from build123d import *

# Parameters (mm, degrees)
BOSS_EXTRUDE1_DEPTH = 9.525
SKETCH3_RX          = 7.62
SKETCH3_RY          = 6.35
CUT_EXTRUDE1_DEPTH  = 35.077675977
SKETCH4_W           = 6.35
SKETCH4_H           = 15.24
BOSS_EXTRUDE2_DEPTH = 3.175
SKETCH5_R           = 3.175
BOSS_EXTRUDE3_DEPTH = 3.175
SKETCH6_W           = 6.35
SKETCH6_H           = 3.81
CUT_EXTRUDE2_DEPTH  = 19.05


with BuildPart() as part:
    # Sketch1 → Boss-Extrude1 (new body, symmetric)
    with BuildSketch(Plane.XY):
        Polygon((-12.7, 12.7), (12.7, 0), (12.7, -12.7), (-12.7, -12.7), align=None)
    extrude(amount=BOSS_EXTRUDE1_DEPTH, both=True)

    # Sketch3 → Cut-Extrude1 (cut, through all)
    with BuildSketch(Plane(origin=(-15.24, 7.62, 0), x_dir=(0, 0, -1), z_dir=(-0.894427191, 0.447213595, 0))):
        with Locations(Location((0, -5.679612663), (0, 0, 0))):
            Ellipse(SKETCH3_RX, SKETCH3_RY)
    extrude(amount=-CUT_EXTRUDE1_DEPTH, mode=Mode.SUBTRACT)

    # Sketch4 → Boss-Extrude2 (add)
    with BuildSketch(Plane.XY.offset(9.525)):
        with Locations((0, -5.08)):
            Rectangle(SKETCH4_W, SKETCH4_H)
    boss_extrude2 = extrude(amount=BOSS_EXTRUDE2_DEPTH)

    # Sketch5 → Boss-Extrude3 (add)
    with BuildSketch(Plane.XY.offset(3.175)):
        with BuildLine():
            Line((-6.35, -12.7), (-6.35, -18.415))
            ThreePointArc((-6.35, -18.415), (0, -24.765), (6.35, -18.415))
            Line((6.35, -18.415), (6.35, -12.7))
            Line((6.35, -12.7), (-6.35, -12.7))
        make_face()
        with Locations((0, -18.415)):
            Circle(SKETCH5_R, mode=Mode.SUBTRACT)
    boss_extrude3 = extrude(amount=BOSS_EXTRUDE3_DEPTH)

    # Mirror1: Boss-Extrude2, Boss-Extrude3 across plane
    add(boss_extrude2.mirror(Plane.XY))
    add(boss_extrude3.mirror(Plane.XY))

    # Sketch6 → Cut-Extrude2 (cut)
    with BuildSketch(Plane(origin=(12.7, 0, 0), x_dir=(0, 0, -1), z_dir=(1, 0, 0))):
        with Locations((0, -10.795)):
            Rectangle(SKETCH6_W, SKETCH6_H)
    extrude(amount=-CUT_EXTRUDE2_DEPTH, mode=Mode.SUBTRACT)


solid = part.part
Geometry check sheet. Reference: the model listing, model coordinates, mm. A direction names the side the tool comes from. Give positions to 0.01 mm unless a question says otherwise; leave off trailing zeros. Loops run counter-clockwise (first coordinate to the right, second up) from the corner with the lowest first, then second, coordinate; pieces in that order, holes last.
(1) Section check A-A on y = -20.5. Record the cut outline in (x, z) (3 decimals), then the cut area to 3 significant figures.
From the geometry:
outline: (-5.998, -6.35) - (-2.394, -6.35) - (-2.394, -3.175) - (-5.998, -3.175) - close; (-5.998, 3.175) - (-2.394, 3.175) - (-2.394, 6.35) - (-5.998, 6.35) - close; (2.394, -6.35) - (5.998, -6.35) - (5.998, -3.175) - (2.394, -3.175) - close; (2.394, 3.175) - (5.998, 3.175) - (5.998, 6.35) - (2.394, 6.35) - close
area: 45.8 mm2
(2) Section check D-D on y = -12. Record the cut outline in (x, z) (3 decimals).
From the geometry:
outline: (-12.7, -9.525) - (-3.175, -9.525) - (-3.175, -12.7) - (3.175, -12.7) - (3.175, -9.525) - (12.7, -9.525) - (12.7, -3.175) - (-6.35, -3.175) - (-6.35, 3.175) - (12.7, 3.175) - (12.7, 9.525) - (3.175, 9.525) - (3.175, 12.7) - (-3.175, 12.7) - (-3.175, 9.525) - (-12.7, 9.525) - close
(3) Release check for a two-part mould opening along Z. For faces 5 (the flat face through (1, -15, -3.175)), 6 (the flat face through (-12.7, -3, 0)), 7 (the flat face through (-3, -20, -6.35)) record: released by +Z, released by -Z, zero draft, split by the parting line, or undercut.
From the geometry:
face 5: undercut
face 6: zero draft
face 7: released by -Z
(4) Thickness scan on L1, parallel to Z at x = -3, y = -11.5 (3 decimals); L2, parallel to X at y = -9, z = -10.5 (3 decimals); L3, parallel to Z at x = 11, y = -5 (3 decimals). Record the ranges inside material, lowest first.
From the geometry:
L1: z = -12.7 to -3.175, 3.175 to 12.7
L2: x = -3.175 to 3.175
L3: z = -9.525 to -4.317, 4.317 to 9.525
(5) Section check C-C on z = 8.75. Record the cut outline in (x, y).
From the geometry:
outline: (-12.7, -12.7) - (12.7, -12.7) - (12.7, 0) - (-12.7, 12.7) - close
(6) Depth check by flat-ended pin: pin 1 Ø5 at (x, y) = (4.5, -20.5) entering from +Z; pin 2 Ø3.5 at (y, z) = (-8, 10.5) entering from -X; pin 3 Ø1 at (y, z) = (-17, 4.5) entering from -X; pin 4 Ø3 at (y, z) = (-10.5, -0.5) entering from +X. Enter the tip coordinate at first touch or a pass-through.
From the geometry:
pin 1: stops at z = 6.35
pin 2: stops at x = -12.7
pin 3: stops at x = -6.35
pin 4: stops at x = -6.35
(7) Set-up check for faces 1 (the flat face through (-3.175, -5, 11)), 2 (the flat face through (6.35, -16, -5)), 3 (the flat face through (-3.175, -5, -11)), 4 (the flat face through (-3, -20, 6.35)): record each of +Z, -Z, +X, -X, +Y, -Y from which the full face is reachable in a straight line by a thin tool's end or side.
From the geometry:
face 1: +Z, -X, +Y, -Y
face 2: +Z, -Z, +X, -Y
face 3: -Z, -X, +Y, -Y
face 4: +Z, +X, -X, -Y
(8) Section check B-B on x = 0. Count the separate pieces of the cut face and the enclosed holes in it, then the cut area to 3 significant figures.
From the geometry:
separate pieces: 3
enclosed holes: 0
area: 387 mm2
